from build123d import *

# Parameters (mm, degrees)
F1_DEPTH = 21.43125
F2_R     = 9.525
F3_DEPTH = 50.8
F4_R     = 4.445
F4_R_2   = 1.5875
F5_DEPTH = 42.8635


with BuildPart() as f1:
    # F0 (on Right) → F1 (new body, symmetric)
    with BuildSketch(Plane.YZ):
        Polygon((-152.4, 69.85), (-152.4, 0), (152.4, 0), (152.4, 19.05), align=None)
    extrude(amount=F1_DEPTH, both=True)

    # F2 (on face) → F3 (cut)
    with BuildSketch(Plane.XZ.offset(152.4)):
        with Locations((0, 34.925)):
            Circle(F2_R)
    extrude(amount=-F3_DEPTH, mode=Mode.SUBTRACT)

    # F4 (on face) → F5 (intersect, through all)
    with BuildSketch(Plane.YZ.offset(21.43125)):
        with BuildLine():
            add(Edge.make_bspline(
                [(-152.4, 69.85), (-121.3656988164, 61.9505317028), (-90.3313976582, 54.0510634121), (-68.8373446816, 43.905343877)],
                knots=[0, 0, 0, 0, 0.298244377, 0.298244377, 0.298244377, 0.298244377], degree=3))
            Line((-152.4, 69.85), (-152.4, 0))
            Line((-152.4, 0), (89.0480875969, 0))
            add(Edge.make_bspline(
                [(11.0622523739, 26.2030381672), (33.9802557949, 23.9980037311), (61.5141716843, 11.9990018706), (89.0480875969, 0)],
                knots=[0.7108019534, 0.7108019534, 0.7108019534, 0.7108019534, 1, 1, 1, 1], degree=3))
            add(Edge.make_bspline(
                [(-31.9974124432, 26.681477204), (-19.2539773306, 24.1221974468), (-4.6688570157, 27.4575486936), (11.0622523353, 26.2030381709)],
                knots=[0.5026616476, 0.5026616476, 0.5026616476, 0.5026616476, 0.67191681, 0.67191681, 0.67191681, 0.67191681], degree=3))
            add(Edge.make_bspline(
                [(-36.899590382, 27.9662974151), (-35.2882031733, 27.4415892282), (-33.6596662635, 27.0073672393), (-31.9974124719, 26.6814772096)],
                knots=[0.4733294563, 0.4733294563, 0.4733294563, 0.4733294563, 0.501572538, 0.501572538, 0.501572538, 0.501572538], degree=3))
            add(Edge.make_bspline(
                [(-68.8373446465, 43.9053438604), (-56.8790512682, 38.1190372354), (-47.2945707385, 31.3048888776), (-36.899590382, 27.9662974151)],
                knots=[0.3381802775, 0.3381802775, 0.3381802775, 0.3381802775, 0.4805951467, 0.4805951467, 0.4805951467, 0.4805951467], degree=3))
        make_face()
        with Locations((-123.747177422, 14.2507199198)):
            Circle(F4_R, mode=Mode.SUBTRACT)
        with Locations((26.8527399749, 9.525)):
            Circle(F4_R_2, mode=Mode.SUBTRACT)
    extrude(amount=-F5_DEPTH, mode=Mode.INTERSECT)


solid = f1.part
Verification items for the finished model (mm, model axes). A direction names the side the tool comes from. Give positions to 0.01 mm unless a question says otherwise; leave off trailing zeros. Use one line per item in the form item = value. Start each with the question number.
Q1. Scan lines: line 1 along Z through (x, y) = (0, -111.5); line 2 along Z through (x, y) = (0, -114); line 3 along Y through (x, z) = (9, 9). Record each from-to range of solid material in increasing order. Write a range as [from, to].
Q2. Mould release check, pull along Z, two halves, no side actions. Record for faces 3 (the flat face through (-21.431, -60, 28)), 4 (the flat face through (0, -33, 0)), 5 (the flat face through (0, -101.6, 35)): +Z half, -Z half, draft (parallel to the pull), parting line (faces both ways), or undercut.
Q3. Access from +Z, -Z, +X, -X, +Y, -Y to the whole of each face (thin tool, end or side, straight path). Record for faces 1 (the flat face through (5.1, -152.4, 43.2)), 2 (the cylindrical face through (-1.24, -127.36, 44.37)).
Q4. Go/stop test with flat-tipped pins: pin 1 Ø15 at (x, z) = (0, 33.5) entering from -Y; pin 2 Ø10 at (x, z) = (5.5, 52.5) entering from +Y; pin 3 Ø10 at (x, y) = (1.5, 55.5) entering from +Z. Record where each tip stops, or that it passes through.
Q5. Section check A-A (x = 0). Count the separate pieces of the cut face and the enclosed holes in it, then the cut area to 3 significant figures.
Evaluation:
q1.line_1 = [0, 25.4], [44.45, 59.02]
q1.line_2 = [0, 25.4], [44.45, 59.73]
q1.line_3 = [-152.4, 25.35], [28.35, 68.1]
q2.face_3 = draft
q2.face_4 = -Z half
q2.face_5 = undercut
q3.face_1 = +Z, -Z, +X, -X, -Y
q3.face_2 = -Y
q4.pin_1 = -101.6
q4.pin_2 = -77.06
q4.pin_3 = 15.98
q5.separate_pieces = 1
q5.enclosed_holes = 2
q5.area = 7,400 mm2
